Verification items for this drawing (mm, ordinates from the low corner). A direction names the side the tool comes from. Round coordinates to 2 decimals unless told otherwise and drop trailing zeros. Order: outer loops, then holes, each group sorted by start corner. A loop starts at its lowest first (then second) coordinate and runs counter-clockwise, first axis right, second up.
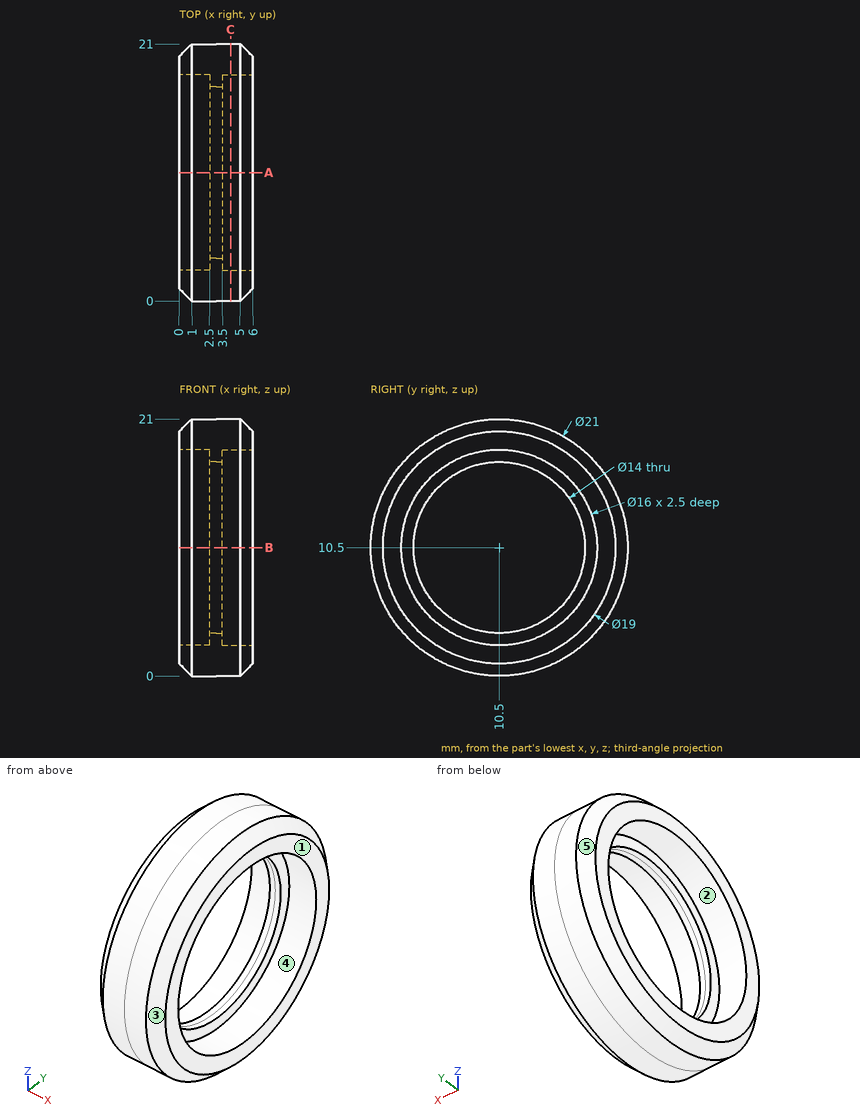
Item 1: Sectioned sample at A-A (y = 10.5). Record the cut outline in (x, z), and give its area (3 significant figures).
Answer:
outline: (0, 1) - (1, 0) - (5, 0) - (6, 1) - (6, 2.5) - (3.5, 2.5) - (3.5, 3.5) - (2.5, 3.5) - (2.5, 2.5) - (0, 2.5) - close; (0, 18.5) - (2.5, 18.5) - (2.5, 17.5) - (3.5, 17.5) - (3.5, 18.5) - (6, 18.5) - (6, 20) - (5, 21) - (1, 21) - (0, 20) - close
area: 30.0 mm2
Item 2: Sectioned sample at C-C (x = 4.2). Record the cut outline in (y, z).
Answer:
outline: circle Ø21 at (10.5, 10.5); hole circle Ø16 at (10.5, 10.5)
Item 3: Release check for a two-part mould opening along Z. For the marked faces 1, 2 and 3 record: released by +Z, released by -Z, zero draft, split by the parting line, or undercut.
Answer:
face 1: zero draft
face 2: undercut
face 3: split by the parting line
Item 4: Go/stop test with flat-tipped pins: P1, Ø5, axis at y = 5, z = 16.5, coming from the -X side; P2, Ø1, axis at x = 1.5, y = 8.5, coming from the +Z side; P3, Ø2, axis at x = 2.5, z = 13.5, coming from the -Y side; P4, Ø1.5, axis at x = 5, y = 6, coming from the -Z side. Record where each tip stops, or that it passes through.
Answer:
P1: stops at x = 0
P2: stops at z = 20.89
P3: stops at y = 0.19
P4: stops at z = 0.69
Item 5: Access from +Z, -Z, +X, -X, +Y, -Y to the whole of each face (thin tool, end or side, straight path). Record for the marked faces 4 and 5.
Answer:
face 4: +X
face 5: -X
Item 6: Scan lines: line 1 along Z through (x, y) = (2.75, 10.5); line 2 along Y through (x, z) = (1.6, 10.75). Record each from-to range of solid material in increasing order.
Answer:
line 1: z = 0 to 3.5, 17.5 to 21
line 2: y = 0 to 2.5, 18.5 to 21
